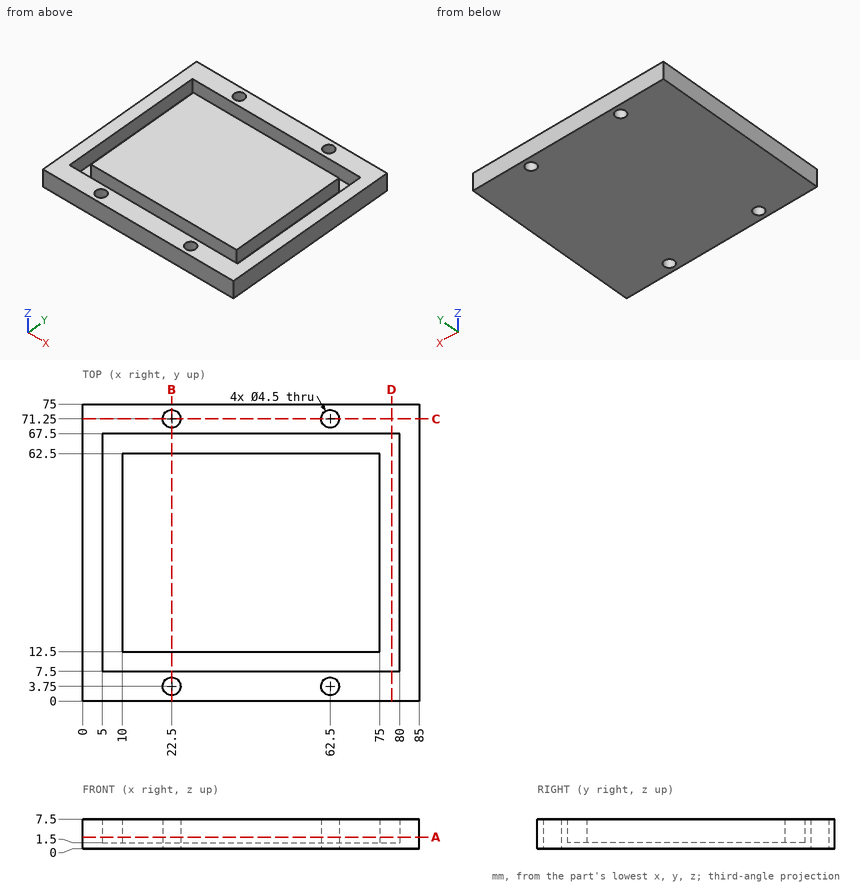
Answer from the drawing. Dimensions are ordinates in mm from the lowest x, y and z of the part. Give positions to 0.01 mm unless a question says otherwise; leave off trailing zeros. Order: outer loops, then holes, each group sorted by start corner. A loop starts at its lowest first (then second) coordinate and runs counter-clockwise, first axis right, second up. Notation, with made-up numbers: (-0.5, 74.5) -> (43.5, 74.5) arc R9 cw to (43.5, 78.5) -> close; hole circle Ø11 at (86, 22.25). An arc over 180 degrees is marked (long way). One line per item, written item: value. Start each with the question number.
(1) Straight lines are drawn through the part: L1, parallel to X at y = 71.25, z = 2.75; L2, parallel to Y at x = 10.5, z = 5.5; L3, parallel to Y at x = 22.5, z = 4.25. For each, find the intervals that lie inside material, in ascending order.
(2) Flat-ended cylindrical pins translate along their axes: P1, Ø7, axis at x = 62.5, y = 3.75, coming from the +Z side; P2, Ø4, axis at x = 62.5, y = 71.25, coming from the +Z side. Find the tip coordinate at first contact, or state that the pin passes through.
(3) The part is cut by section B-B (x = 22.5). Determine the outline of the cut face in (y, z).
(4) The part is cut by section A-A (z = 3). Determine the outline of the cut face in (x, y).
(5) The part is cut by section D-D (x = 78). Determine the outline of the cut face in (y, z), and give its area (4 significant figures).
(6) The part is cut by section C-C (y = 71.25). Determine the outline of the cut face in (x, z).
Taken from the geometry:
1. L1: 0 to 20.25, 24.75 to 60.25, 64.75 to 85
1. L2: 0 to 7.5, 12.5 to 62.5, 67.5 to 75
1. L3: 0 to 1.5, 6 to 7.5, 12.5 to 62.5, 67.5 to 69, 73.5 to 75
2. P1: z = 7.5
2. P2: through
3. outline: (0, 0) -> (1.5, 0) -> (1.5, 7.5) -> (0, 7.5) -> close; (6, 0) -> (69, 0) -> (69, 7.5) -> (67.5, 7.5) -> (67.5, 1.5) -> (62.5, 1.5) -> (62.5, 7.5) -> (12.5, 7.5) -> (12.5, 1.5) -> (7.5, 1.5) -> (7.5, 7.5) -> (6, 7.5) -> close; (73.5, 0) -> (75, 0) -> (75, 7.5) -> (73.5, 7.5) -> close
4. outline: (0, 0) -> (85, 0) -> (85, 75) -> (0, 75) -> close; (10, 12.5) -> (75, 12.5) -> (75, 62.5) -> (10, 62.5) -> close; hole (5, 7.5) -> (80, 7.5) -> (80, 67.5) -> (5, 67.5) -> close; hole circle Ø4.5 at (22.5, 3.75); hole circle Ø4.5 at (22.5, 71.25); hole circle Ø4.5 at (62.5, 3.75); hole circle Ø4.5 at (62.5, 71.25)
5. outline: (0, 0) -> (75, 0) -> (75, 7.5) -> (67.5, 7.5) -> (67.5, 1.5) -> (7.5, 1.5) -> (7.5, 7.5) -> (0, 7.5) -> close
5. area: 202.5 mm^2
6. outline: (0, 0) -> (20.25, 0) -> (20.25, 7.5) -> (0, 7.5) -> close; (24.75, 0) -> (60.25, 0) -> (60.25, 7.5) -> (24.75, 7.5) -> close; (64.75, 0) -> (85, 0) -> (85, 7.5) -> (64.75, 7.5) -> close
